```python
from build123d import *

# Parameters (mm, degrees)
SKETCH1_W             = 198
SKETCH1_H             = 108
BOSS_EXTRUDE1_DEPTH   = 40
SKETCH4_W             = 181
SKETCH4_H             = 45
CUT_EXTRUDE2_DEPTH    = 10
CUT_EXTRUDE3_START    = -198
CUT_EXTRUDE3_DEPTH    = 198
BOSS_EXTRUDE11_DEPTH  = 10
CUT_EXTRUDE12_DEPTH   = 198
CUT_EXTRUDE28_DEPTH   = 14.5
CUT_EXTRUDE29_DEPTH   = 14.5
CUT_EXTRUDE40_REACH   = 231.059
SKETCH12_R            = 3.15
CUT_EXTRUDE9_DEPTH    = 230.058944379
SKETCH13_R            = 4.5
CUT_EXTRUDE10_DEPTH   = 16.5
SKETCH14_R            = 4.5
CUT_EXTRUDE11_DEPTH   = 16.5
SKETCH41_R            = 2.9
CUT_EXTRUDE21_DEPTH   = 7
CUT_EXTRUDE22_DEPTH   = 10
CUT_EXTRUDE23_DEPTH   = 10
CUT_EXTRUDE35_DEPTH   = 55.4
CUT_EXTRUDE34_DEPTH   = 55.4
CUT_EXTRUDE36_DEPTH   = 55.4
SKETCH90_R            = 6.1
CUT_EXTRUDE38_DEPTH   = 17
SKETCH96_R            = 2
CUT_EXTRUDE39_DEPTH   = 230.058944379
SKETCH98_R            = 7.5
CUT_EXTRUDE41_DEPTH   = 4
CROQUIS1_W            = 146
CROQUIS1_H            = 68
CORTAR_EXTRUIR1_DEPTH = 15


with BuildPart() as part:
    # Sketch1 → Boss-Extrude1 (new body)
    with BuildSketch(Plane(origin=(0, 0, 0), x_dir=(1, 0, 0), z_dir=(0, 1, 0))):
        with Locations((99, 54)):
            Rectangle(SKETCH1_W, SKETCH1_H)
    extrude(amount=BOSS_EXTRUDE1_DEPTH)

    # Sketch4 → Cut-Extrude2 (cut)
    with BuildSketch(Plane(origin=(0, 0, 0), x_dir=(1, 0, 0), z_dir=(0, 1, 0))):
        with Locations((99, 54)):
            Rectangle(SKETCH4_W, SKETCH4_H)
    extrude(amount=CUT_EXTRUDE2_DEPTH, mode=Mode.SUBTRACT)

    # Sketch5 → Cut-Extrude3 (cut)
    with BuildSketch(Plane(origin=(198, 0, 0), x_dir=(0, 0, -1), z_dir=(1, 0, 0)).offset(CUT_EXTRUDE3_START)):
        Polygon((54, 40), (108, 35.674234207), (108, 40), align=None)
    extrude(amount=CUT_EXTRUDE3_DEPTH, mode=Mode.SUBTRACT)

    # Sketch53 → Boss-Extrude11 (add)
    with BuildSketch(Plane(origin=(0, 10, 0), x_dir=(-1, 0, 0), z_dir=(0, -1, 0))):
        Polygon((-8.5, 51.5), (-8.5, 31.5), (-39.5, 31.5), align=None)
        Polygon((-8.5, 56.5), (-8.5, 76.5), (-39.5, 76.5), align=None)
        Polygon((-158.5, 76.5), (-189.5, 56.5), (-189.5, 76.5), align=None)
        Polygon((-158.5, 31.5), (-189.5, 51.5), (-189.5, 31.5), align=None)
    extrude(amount=BOSS_EXTRUDE11_DEPTH)

    # Sketch18 → Cut-Extrude12 (cut)
    with BuildSketch(Plane(origin=(198, 0, 0), x_dir=(0, 0, -1), z_dir=(1, 0, 0))):
        Polygon((0, 35.674234207), (0, 40), (54, 40), align=None)
    extrude(amount=-CUT_EXTRUDE12_DEPTH, mode=Mode.SUBTRACT)

    # Izq → Cut-Extrude28 (cut)
    with BuildSketch(Plane(origin=(0, 28.012686094, -12.204810084), x_dir=(1, 0, 0), z_dir=(0, 0.9167660546215652, -0.39942458749256926))):
        Polygon((8.5, 48.862182113), (29.5, 70.132603179), (8.5, 70.132603179), align=None)
    cut_extrude28 = extrude(amount=-CUT_EXTRUDE28_DEPTH, mode=Mode.SUBTRACT)

    # Der → Cut-Extrude29 (cut)
    with BuildSketch(Plane(origin=(0, -11.144923858, -4.62106599), x_dir=(1, 0, 0), z_dir=(0, 0.9237421135716327, 0.38301502270043264))):
        Polygon((8.5, 51.290217599), (29.5, 29.097876578), (8.5, 29.097876578), align=None)
    cut_extrude29 = extrude(amount=-CUT_EXTRUDE29_DEPTH, mode=Mode.SUBTRACT)

    # Cut-Extrude40: up to this face of the body (flat: up to its plane)
    cut_extrude40_end = Plane(part.part.faces().sort_by_distance((99, 10, -54))[0])
    # Sketch97 → Cut-Extrude40 (cut, up to the picked face)
    with BuildSketch(Plane(origin=(0, 0, 0), x_dir=(1, 0, 0), z_dir=(0, 1, 0)), mode=Mode.PRIVATE) as cut_extrude40_sk1:
        Polygon((8.5, 57.5), (29.5, 76.5), (158.5, 76.5), (189.5, 56.5), (189.5, 51.5), (158.5, 31.5), (29.5, 31.5), (8.5, 51.5), align=None)
    cut_extrude40_tool1 = split(extrude(cut_extrude40_sk1.sketch, amount=CUT_EXTRUDE40_REACH, mode=Mode.PRIVATE), bisect_by=cut_extrude40_end, keep=Keep.BOTH, mode=Mode.PRIVATE)
    cut_extrude40 = cut_extrude40_tool1.solids().sort_by(Axis((96.82024, 0, -54.014019), (0, 1, 0)))[0]
    add(cut_extrude40, mode=Mode.SUBTRACT)

    # Mirror2: Cut-Extrude28, Cut-Extrude29, Cut-Extrude40 across plane
    add(cut_extrude28.mirror(Plane(origin=(99, 0, 0), x_dir=(0, 0, 1), z_dir=(1, 0, 0))), mode=Mode.SUBTRACT)
    add(cut_extrude29.mirror(Plane(origin=(99, 0, 0), x_dir=(0, 0, 1), z_dir=(1, 0, 0))), mode=Mode.SUBTRACT)
    add(cut_extrude40.mirror(Plane(origin=(99, 0, 0), x_dir=(0, 0, 1), z_dir=(1, 0, 0))), mode=Mode.SUBTRACT)

    # Sketch12 → Cut-Extrude9 (cut, through all)
    with BuildSketch(Plane(origin=(0, 40, 0), x_dir=(1, 0, 0), z_dir=(0, 1, 0))):
        with Locations(Location((19.7, 98.85, 0), (0, 0, 270))):
            Circle(SKETCH12_R)
        with Locations(Location((99.7, 9.15, 0), (0, 0, 270))):
            Circle(SKETCH12_R)
        with Locations(Location((179.7, 9.15, 0), (0, 0, 270))):
            Circle(SKETCH12_R)
        with Locations(Location((19.7, 9.15, 0), (0, 0, 270))):
            Circle(SKETCH12_R)
        with Locations(Location((99.7, 98.85, 0), (0, 0, 270))):
            Circle(SKETCH12_R)
        with Locations(Location((179.7, 98.85, 0), (0, 0, 270))):
            Circle(SKETCH12_R)
    extrude(amount=-CUT_EXTRUDE9_DEPTH, mode=Mode.SUBTRACT)

    # Sketch13 → Cut-Extrude10 (cut)
    with BuildSketch(Plane(origin=(0, 44.04313679, -3.528153602), x_dir=(1, 0, 0), z_dir=(0, 0.9968068124341598, -0.07985097798305206))):
        with Locations(Location((46.5, 91.806513253, 0), (0, 0, 270))):
            Circle(SKETCH13_R)
        with Locations(Location((151.5, 91.806513253, 0), (0, 0, 270))):
            Circle(SKETCH13_R)
    extrude(amount=-CUT_EXTRUDE10_DEPTH, mode=Mode.SUBTRACT)

    # Sketch14 → Cut-Extrude11 (cut)
    with BuildSketch(Plane(origin=(0, 35.212287021, 5.766643233), x_dir=(1, 0, 0), z_dir=(0, 0.9968068124341597, 0.07985097798305243))):
        with Locations(Location((46.5, 18.739607443, 0), (0, 0, 270))):
            Circle(SKETCH14_R)
        with Locations(Location((151.5, 18.739607443, 0), (0, 0, 270))):
            Circle(SKETCH14_R)
    extrude(amount=-CUT_EXTRUDE11_DEPTH, mode=Mode.SUBTRACT)

    # Sketch41 → Cut-Extrude21 (cut)
    with BuildSketch(Plane(origin=(0, 0, 0), x_dir=(1, 0, 0), z_dir=(0, 1, 0))):
        with Locations(Location((139.5, 9, 0), (0, 0, 90))):
            Circle(SKETCH41_R)
        with Locations(Location((139.5, 99, 0), (0, 0, 90))):
            Circle(SKETCH41_R)
    extrude(amount=CUT_EXTRUDE21_DEPTH, mode=Mode.SUBTRACT)

    # Sketch42 → Cut-Extrude22 (cut)
    with BuildSketch(Plane.XY):
        with BuildLine():
            Line((142.3, 12.8), (152, 12.8))
            ThreePointArc((152, 12.8), (153.8, 11), (152, 9.2))
            Line((152, 9.2), (142.3, 9.2))
            ThreePointArc((142.3, 9.2), (140.5, 11), (142.3, 12.8))
        make_face()
    extrude(amount=-CUT_EXTRUDE22_DEPTH, mode=Mode.SUBTRACT)

    # Sketch43 → Cut-Extrude23 (cut)
    with BuildSketch(Plane(origin=(0, 0, -108), x_dir=(-1, 0, 0), z_dir=(0, 0, -1))):
        with BuildLine():
            Line((-55.7, 12.8), (-46, 12.8))
            ThreePointArc((-46, 12.8), (-44.2, 11), (-46, 9.2))
            Line((-46, 9.2), (-55.7, 9.2))
            ThreePointArc((-55.7, 9.2), (-57.5, 11), (-55.7, 12.8))
        make_face()
    extrude(amount=-CUT_EXTRUDE23_DEPTH, mode=Mode.SUBTRACT)

    # Sketch84 → Cut-Extrude35 (cut)
    with BuildSketch(Plane(origin=(0, 44.04313679, -3.528153602), x_dir=(1, 0, 0), z_dir=(0, 0.9968068124341598, -0.07985097798305206))):
        with BuildLine():
            Line((31.7, 54.733528752), (166.7, 54.733528752))
            ThreePointArc((166.7, 54.733528752), (168.467766953, 55.465761799), (169.2, 57.233528752))
            Line((169.2, 57.233528752), (169.2, 72.233528752))
            ThreePointArc((169.2, 72.233528752), (168.467766953, 74.001295705), (166.7, 74.733528752))
            Line((166.7, 74.733528752), (31.7, 74.733528752))
            ThreePointArc((31.7, 74.733528752), (29.932233047, 74.001295705), (29.2, 72.233528752))
            Line((29.2, 72.233528752), (29.2, 57.233528752))
            ThreePointArc((29.2, 57.233528752), (29.932233047, 55.465761799), (31.7, 54.733528752))
        make_face()
    extrude(amount=-CUT_EXTRUDE35_DEPTH, mode=Mode.SUBTRACT)

    # Sketch83 → Cut-Extrude34 (cut)
    with BuildSketch(Plane(origin=(0, 35.446768916, 2.839526304), x_dir=(1, 0, 0), z_dir=(0, 0.9968068124341598, 0.07985097798305245))):
        with BuildLine():
            Line((31.7, 52.921606991), (166.7, 52.921606991))
            ThreePointArc((166.7, 52.921606991), (168.467766953, 52.189373944), (169.2, 50.421606991))
            Line((169.2, 50.421606991), (169.2, 35.421606991))
            ThreePointArc((169.2, 35.421606991), (168.467766953, 33.653840038), (166.7, 32.921606991))
            Line((166.7, 32.921606991), (31.7, 32.921606991))
            ThreePointArc((31.7, 32.921606991), (29.932233047, 33.653840038), (29.2, 35.421606991))
            Line((29.2, 35.421606991), (29.2, 50.421606991))
            ThreePointArc((29.2, 50.421606991), (29.932233047, 52.189373944), (31.7, 52.921606991))
        make_face()
    extrude(amount=-CUT_EXTRUDE34_DEPTH, mode=Mode.SUBTRACT)

    # Sketch85 → Cut-Extrude36 (cut)
    with BuildSketch(Plane(origin=(0, 40, 0), x_dir=(1, 0, 0), z_dir=(0, 1, 0))):
        Polygon((0, 101.9), (6.1, 108), (0, 108), align=None)
        Polygon((0, 0), (6.1, 0), (0, 6.1), align=None)
        Polygon((198, 6.1), (191.9, 0), (198, 0), align=None)
        Polygon((198, 108), (191.9, 108), (198, 101.9), align=None)
    extrude(amount=-CUT_EXTRUDE36_DEPTH, mode=Mode.SUBTRACT)

    # Sketch90 → Cut-Extrude38 (cut)
    with BuildSketch(Plane(origin=(0, 40, 0), x_dir=(1, 0, 0), z_dir=(0, 1, 0))):
        with Locations(Location((19.7, 9.15, 0), (0, 0, 270))):
            Circle(SKETCH90_R)
        with Locations(Location((99.7, 9.15, 0), (0, 0, 270))):
            Circle(SKETCH90_R)
        with Locations(Location((179.7, 9.15, 0), (0, 0, 270))):
            Circle(SKETCH90_R)
        with Locations(Location((99.7, 98.85, 0), (0, 0, 270))):
            Circle(SKETCH90_R)
        with Locations(Location((179.7, 98.85, 0), (0, 0, 270))):
            Circle(SKETCH90_R)
        with Locations(Location((19.7, 98.85, 0), (0, 0, 270))):
            Circle(SKETCH90_R)
    extrude(amount=-CUT_EXTRUDE38_DEPTH, mode=Mode.SUBTRACT)

    # Sketch96 → Cut-Extrude39 (cut, through all)
    with BuildSketch(Plane(origin=(0, 0, 0), x_dir=(1, 0, 0), z_dir=(0, 1, 0))):
        with Locations(Location((15.45, 54, 0), (0, 0, 180))):
            Circle(SKETCH96_R)
        with Locations((185, 54)):
            Circle(SKETCH96_R)
    extrude(amount=CUT_EXTRUDE39_DEPTH, mode=Mode.SUBTRACT)

    # Sketch98 → Cut-Extrude41 (cut)
    with BuildSketch(Plane(origin=(0, 40, 0), x_dir=(1, 0, 0), z_dir=(0, 1, 0))):
        with Locations(Location((185, 54, 0), (0, 0, 270))):
            Circle(SKETCH98_R)
        with Locations(Location((15.45, 54, 0), (0, 0, 270))):
            Circle(SKETCH98_R)
    extrude(amount=-CUT_EXTRUDE41_DEPTH, mode=Mode.SUBTRACT)

    # Croquis1 → Cortar-Extruir1 (cut)
    with BuildSketch(Plane(origin=(0, 40, 0), x_dir=(1, 0, 0), z_dir=(0, 1, 0))):
        with Locations((99, 54)):
            Rectangle(CROQUIS1_W, CROQUIS1_H)
    extrude(amount=-CORTAR_EXTRUIR1_DEPTH, mode=Mode.SUBTRACT)


solid = part.part
```
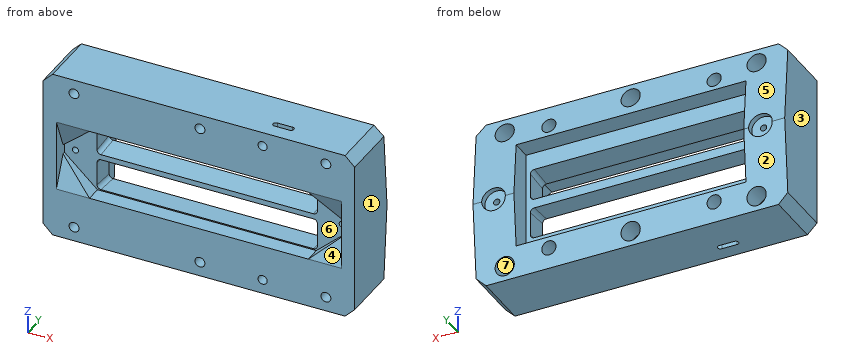
For this review, take the finished solid that the model builds, in its own axes (mm). Face numbers are marked on the shaded views. A direction names the side the tool comes from. Round coordinates to 2 decimals unless told otherwise and drop trailing zeros. Write each loop counter-clockwise with the first axis right and the second up, starting at its lowest first coordinate (ties: lowest second). Pieces come first, ordered by that corner, then holes. Notation, with made-up numbers: (-11.75, -12) -> (0.25, -12) arc R23 cw to (0.25, 18) -> close; hole circle Ø10 at (51, 46.25). An arc over 180 degrees is marked (long way). One line per question, with ' | ' between items. Start each with the question number.
(1) Insertion check: P1, Ø22.5, axis at x = 118.5, z = -60.5, coming from the -Y side; P2, Ø12, axis at y = 31, z = -58.5, coming from the -X side; P3, Ø3, axis at x = 146, z = -6.5, coming from the +Y side; P4, Ø16, axis at x = 179.7, z = -98.85, coming from the +Y side. Each pin has a flat end and moves straight along its axis. Give the tip position at first contact, or say it passes through.
(2) Add section B-B, the plane y = 3. Give the number of separate pieces and of enclosed holes in the cut face, plus the area to 3 significant figures.
(3) For line 1 along Z through (x, y) = (19.7, 32.5); line 2 along Z through (x, y) = (99.7, 28.25); line 3 along Z through (x, y) = (179.7, 10.25), list the stretches that pass through material, from the lowest coordinate up. Write a range as from..to.
(4) Add section D-D, the plane z = -25.5. Write out the cut boundary in (x, y), plus the area to 3 significant figures.
(5) Tool access review of the marked faces 5, 6 and 7: name each direction out of +Z, -Z, +X, -X, +Y, -Y from which nothing blocks a thin tool from reaching the whole face with its end or side.
(6) Add section A-A, the plane x = 86.5. Write out the cut boundary in (y, z).
(7) Mouldability with a two-part tool opening along X and no side actions: class the marked faces 1, 2, 3 and 4 as released by +X, released by -X, zero draft, split by the parting line, or undercut.
Answer list:
1) P1: y = 10 | P2: x = 0 | P3: y = 36.32 | P4: y = 37.05
2) separate pieces: 1 | enclosed holes: 9 | area: 13,400 mm²
3) line 1: -108..-104.95, -92.75..-15.25, -3.05..0 | line 2: -108..-104.95, -92.75..-88, -20..-15.25, -3.05..0 | line 3: -108..-102, -95.7..-12.3, -6..0
4) outline: (0, 0) -> (198, 0) -> (198, 37.72) -> (172, 37.72) -> (172, 25) -> (26, 25) -> (26, 37.72) -> (0, 37.72) -> close | area: 5,610 mm²
5) face 5: +Z, +X, -X, +Y | face 6: -Y | face 7: +Y
6) outline: (0, -108) -> (35.67, -108) -> (37.28, -88) -> (25, -88) -> (25, -76.98) -> (10, -75.77) -> (10, -76.5) -> (0, -76.5) -> close; (0, -31.5) -> (10, -31.5) -> (10, -32.23) -> (25, -31.02) -> (25, -20) -> (37.28, -20) -> (35.67, 0) -> (0, 0) -> close; (10, -55.71) -> (25, -56.91) -> (25, -51.09) -> (10, -52.29) -> close
7) face 1: released by +X | face 2: zero draft | face 3: released by -X | face 4: undercut
